```python
from build123d import *

# Parameters (mm, degrees)
SKETCH1_R           = 1.75
BOSS_EXTRUDE1_DEPTH = 4.5
BOSS_EXTRUDE2_START = -4.5
BOSS_EXTRUDE2_DEPTH = 4.5


with BuildPart() as part:
    # Sketch1 → Boss-Extrude1 (new body)
    with BuildSketch(Plane.XY):
        with BuildLine():
            ThreePointArc((-11, 5), (-16, 0), (-11, -5))
            Line((-11, -5), (11.000000019, -5))
            ThreePointArc((11.000000019, -5), (16, 9e-09), (11, 5))
            Line((11, 5), (-11, 5))
        make_face()
        with Locations((-11, 0)):
            Circle(SKETCH1_R, mode=Mode.SUBTRACT)
        with Locations((11, 0)):
            Circle(SKETCH1_R, mode=Mode.SUBTRACT)
    extrude(amount=BOSS_EXTRUDE1_DEPTH)

    # Sketch2 → Boss-Extrude2 (add)
    with BuildSketch(Plane.XY.offset(4.5).offset(BOSS_EXTRUDE2_START)):
        with BuildLine():
            Line((47.182162457, 10.03), (45.167162457, 13.485397951))
            add(Edge.make_bspline(
                [(0, 5), (22.415618243, 10.14564432), (45.167162457, 13.485397951)],
                knots=[0, 0, 0, 1, 1, 1], degree=2))
            Line((0, 5), (11, 5))
            ThreePointArc((11, 5), (16, 0), (11, -5))
            Line((11, -5), (13.99, -5))
            Line((13.99, -5), (20.61, -1.48))
            add(Edge.make_bspline(
                [(40.271366555, 6), (32.419293016, 6.4877302), (27.171947838, 2.009132385), (20.61, -1.48)],
                knots=[0, 0, 0, 0, 1, 1, 1, 1], degree=3))
            Line((40.271366555, 6), (47.182162457, 10.03))
        make_face()
    extrude(amount=BOSS_EXTRUDE2_DEPTH)


solid = part.part
```
Source: CAD feature listing. Evaluate the final solid. Frame: model axes, mm. A direction names the side the tool comes from. Round coordinates to 2 decimals unless told otherwise and drop trailing zeros. Write each loop counter-clockwise with the first axis right and the second up, starting at its lowest first coordinate (ties: lowest second). Pieces come first, ordered by that corner, then holes. Notation, with made-up numbers: M 22,48.5 L 36,48.5 A20 cw 36,64.5 Z; hole C 64,3.25 d7. An arc over 180 degrees is marked long. Answer as a JSON object with one key per item and string values. Group by question number.
(1) Section query A-A on z = 0.8. State how many separate pieces and enclosed holes the cut face has, then the cut area to 3 significant figures.
(2) Reachability of faces 4 (the flat face through (-5, 5, 2)), 5 (the flat face through (17.254, -3.265, 2.218)) from +Z, -Z, +X, -X, +Y, -Y: full face, straight path, thin tool, end or side. Return the list, or none.
(3) Mould query, pull axis X, two halves, no side actions, for faces 1 (the flat face through (1, -5, 2)), 2 (the flat face through (46.19, 11.73, 2.22)), 3 (the cylindrical face through (12.669, 0.526, 2.218)). Classes: +X half, -X half, draft (parallel to the pull), parting line (faces both ways), or undercut.
(4) Ray query, line 1 (Y direction, x = -11, z = 2.2); line 2 (Y direction, x = 11, z = 1.9); line 3 (X direction, y = 1.25, z = 0.7). Return the intervals inside material, ascending. Write a range as [from, to].
(5) Section query B-B on x = -7. Output: boundary loops of the cut face in (y, z).
(6) First-contact query: pin 1 (1.5 mm diameter, centred on x = 25.5, z = 1.5, fed in from +Y); pin 2 (8 mm diameter, centred on x = 25.5, y = 10.5, fed in from +Z). Flat tips, straight axial feed; report the tip coordinate or a pass-through.
Computed values:
{
 "1": {"separate pieces": "1", "enclosed holes": "2", "area": "555 mm^2"},
 "2": {"face 4": "+Z, -Z, -X, +Y", "face 5": "+Z, -Z, +X, -Y"},
 "3": {"face 1": "draft", "face 2": "+X half", "face 3": "undercut"},
 "4": {"line 1": "[-5, -1.75], [1.75, 5]", "line 2": "[-5, -1.75], [1.75, 7.41]", "line 3": "[-15.84, -12.22], [-9.78, 9.78], [12.22, 25.38]"},
 "5": {"outline": "M -5,0 L 5,0 L 5,4.5 L -5,4.5 Z"},
 "6": {"pin 1": "y = 10.39", "pin 2": "z = 4.5"}
}
